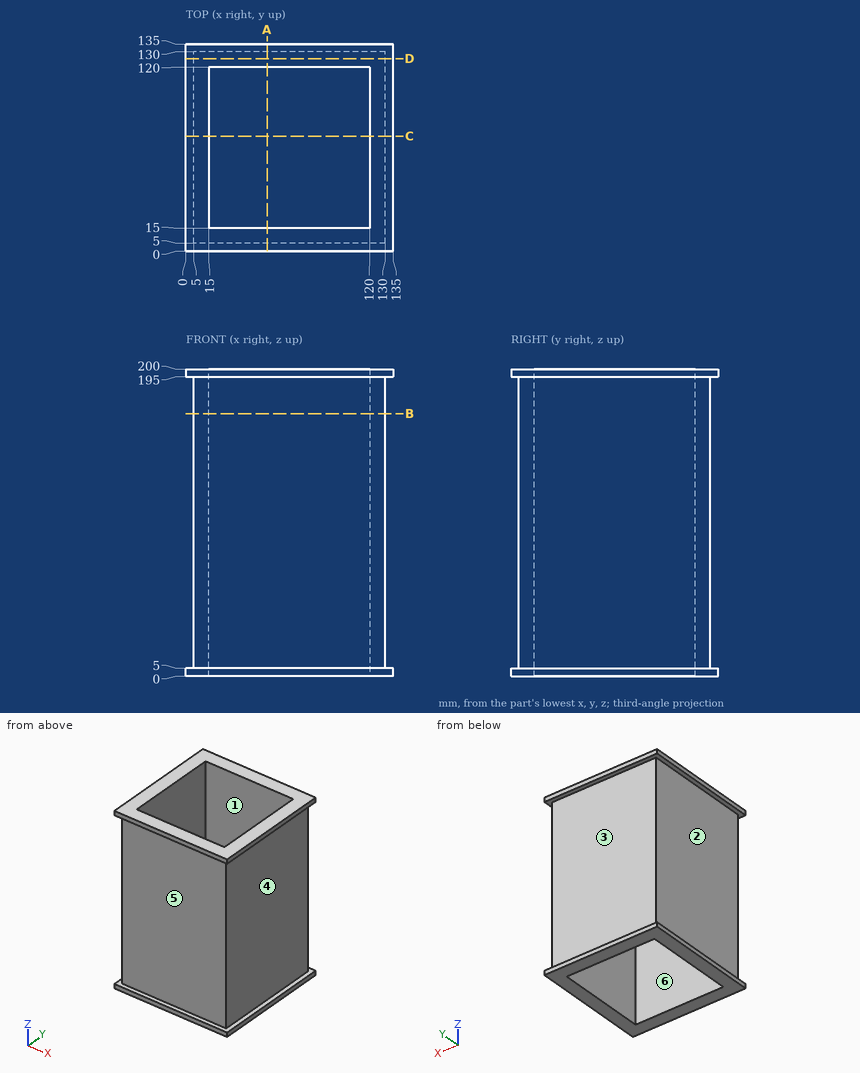
Check sheet for the drawn part. Datum: minimum x, y, z corner. Units: mm. A direction names the side the tool comes from. Round coordinates to 2 decimals unless told otherwise and drop trailing zeros. Write each loop counter-clockwise with the first axis right and the second up, starting at its lowest first coordinate (ties: lowest second). Pieces come first, ordered by that corner, then holes. Notation, with made-up numbers: (-18, 54) -> (11, 54) arc R29 cw to (11, 75) -> close; hole circle Ø5 at (-36, -10.75). An arc over 180 degrees is marked (long way). Write each question's results on one line, items separated by ' | '. Start each with the question number.
1. Material ranges on probe 1 along X at (y, z) = (24.5, 109); probe 2 along X at (y, z) = (10.5, 136.5), recorded low to high. Write a range as from..to.
2. Depth check by flat-ended pin: P1, Ø5, axis at y = 58.5, z = 110.5, coming from the +X side; P2, Ø1.5, axis at x = 13.5, z = 26, coming from the -Y side; P3, Ø2, axis at x = 33.5, z = 86.5, coming from the +Y side; P4, Ø8, axis at x = 117.5, y = 53.5, coming from the -Z side. Enter the tip coordinate at first touch or a pass-through.
3. Cross-section at B-B (z = 171). Enter the section's corners in (x, y).
4. Cross-section at D-D (y = 125.5). Enter the section's corners in (x, z).
5. Cross-section at A-A (x = 53). Enter the section's corners in (y, z), then the cut area to 3 significant figures.
6. Draft check along Z on the marked faces 1 and 2. Enter one of: +Z half, -Z half, draft (parallel to the pull), parting line (faces both ways), or undercut.
7. Set-up check for the marked faces 3, 4, 5 and 6: record each of +Z, -Z, +X, -X, +Y, -Y from which the full face is reachable in a straight line by a thin tool's end or side.
Solutions:
1) probe 1: x = 5..15, 120..130 | probe 2: x = 5..130
2) P1: stops at x = 130 | P2: stops at y = 5 | P3: stops at y = 130 | P4: stops at z = 0
3) outline: (5, 5) -> (130, 5) -> (130, 130) -> (5, 130) -> close; hole (15, 15) -> (120, 15) -> (120, 120) -> (15, 120) -> close
4) outline: (0, 0) -> (135, 0) -> (135, 5) -> (130, 5) -> (130, 195) -> (135, 195) -> (135, 200) -> (0, 200) -> (0, 195) -> (5, 195) -> (5, 5) -> (0, 5) -> close
5) outline: (0, 0) -> (15, 0) -> (15, 200) -> (0, 200) -> (0, 195) -> (5, 195) -> (5, 5) -> (0, 5) -> close; (120, 0) -> (135, 0) -> (135, 5) -> (130, 5) -> (130, 195) -> (135, 195) -> (135, 200) -> (120, 200) -> close | area: 4,100 mm2
6) face 1: draft | face 2: undercut
7) face 3: +X, -X, +Y | face 4: +X, +Y, -Y | face 5: +X, -X, -Y | face 6: +Z, -Z
